```python
from build123d import *

# Parameters (mm, degrees)
SKETCH1_W           = 76.2
SKETCH1_H           = 9.525
SKETCH1_R           = 3.175
BOSS_EXTRUDE1_DEPTH = 12.7
CUT_EXTRUDE1_REACH  = 803.818
SKETCH2_R           = 2.6035


with BuildPart() as part:
    # Sketch1 → Boss-Extrude1 (new body)
    with BuildSketch(Plane(origin=(0, 788.156140976, 0), x_dir=(1, 0, 0), z_dir=(0, 1, 0))):
        with Locations((0, 58.7375)):
            Rectangle(SKETCH1_W, SKETCH1_H)
        with Locations(Location((-20.32, 58.7375, 0), (0, 0, 270))):
            Circle(SKETCH1_R, mode=Mode.SUBTRACT)
        with Locations(Location((20.32, 58.7375, 0), (0, 0, 90))):
            Circle(SKETCH1_R, mode=Mode.SUBTRACT)
    extrude(amount=BOSS_EXTRUDE1_DEPTH)

    # Sketch2 → Cut-Extrude1 (cut, up to next)
    with BuildSketch(Plane(origin=(0, 0, -63.5), x_dir=(-1, 0, 0), z_dir=(0, 0, -1)), mode=Mode.PRIVATE) as cut_extrude1_sk1:
        with Locations((30.1625, 794.506140976)):
            Circle(SKETCH2_R)
    cut_extrude1_tool1 = extrude(cut_extrude1_sk1.sketch, amount=-CUT_EXTRUDE1_REACH, mode=Mode.PRIVATE) & part.part
    # Sketch2 → Cut-Extrude1 (cut, up to next)
    with BuildSketch(Plane(origin=(0, 0, -63.5), x_dir=(-1, 0, 0), z_dir=(0, 0, -1)), mode=Mode.PRIVATE) as cut_extrude1_sk2:
        with Locations((-30.1625, 794.506140976)):
            Circle(SKETCH2_R)
    cut_extrude1_tool2 = extrude(cut_extrude1_sk2.sketch, amount=-CUT_EXTRUDE1_REACH, mode=Mode.PRIVATE) & part.part
    add(cut_extrude1_tool1.solids().sort_by_distance((-30.1625, 794.506141, -63.5))[0], mode=Mode.SUBTRACT)
    add(cut_extrude1_tool2.solids().sort_by_distance((30.1625, 794.506141, -63.5))[0], mode=Mode.SUBTRACT)


solid = part.part
```
Input: part model. Units: mm. Frame: model coordinates. Give positions to 0.01 mm unless a question says otherwise; leave off trailing zeros. Order: outer loops, then holes, each group sorted by start corner. A loop starts at its lowest first (then second) coordinate and runs counter-clockwise, first axis right, second up. Notation, with made-up numbers: (81.5, 64.25) - (91.5, 64.25) arc R26 ccw to (91.5, 92.25) - close; hole circle Ø3 at (51.5, -10.75). An arc over 180 degrees is marked (long way). Use a Markdown table: item, result.
(1) Line query: line 1 (X direction, y = 793.5, z = -56.5); line 2 (X direction, y = 795.75, z = -55); line 3 (X direction, y = 789.25, z = -61.25). Output: solid intervals per line, ascending. Write a range as from..to.
Computed values:
| item | result |
|---|---|
| line 1 | x = -38.1..-32.56, -27.76..-22.57, -18.07..18.07, 22.57..27.76, 32.56..38.1 |
| line 2 | x = -38.1..-32.45, -27.88..27.88, 32.45..38.1 |
| line 3 | x = -38.1..-22.26, -18.38..18.38, 22.26..38.1 |
(2) Pin query (flat end, axial travel): pin 1 (4 mm diameter, centred on x = 30.16, y = 794.51, fed in from +Z) (3 decimals). Return the tip coordinate at first contact, or that it passes through.
Computed values:
| item | result |
|---|---|
| pin 1 | passes through |
(3) Section query A-A (x = 20.32). Output: boundary loops of the cut face in (y, z) (1 decimal), then the cut area to 3 significant figures.
Computed values:
| item | result |
|---|---|
| outline | (788.2, -63.5) - (800.9, -63.5) - (800.9, -61.9) - (788.2, -61.9) - close; (788.2, -55.6) - (800.9, -55.6) - (800.9, -54) - (788.2, -54) - close |
| area | 40.3 mm2 |
(4) Draft query along Y for faces 1 (the flat face through (-1, 800.856, -59)), 2 (the cylindrical face through (30.727, 791.965, -58.804)), 3 (the flat face through (-38.1, 794, -59)). Return one class per face: released by +Y, released by -Y, zero draft, split by the parting line, or undercut.
Computed values:
| item | result |
|---|---|
| face 1 | released by +Y |
| face 2 | undercut |
| face 3 | zero draft |
(5) Section query B-B (z = -58.5). Output: boundary loops of the cut face in (x, y).
Computed values:
| item | result |
|---|---|
| outline | (-38.1, 788.16) - (-23.49, 788.16) - (-23.49, 800.86) - (-38.1, 800.86) - close; (-17.15, 788.16) - (17.15, 788.16) - (17.15, 800.86) - (-17.15, 800.86) - close; (23.49, 788.16) - (38.1, 788.16) - (38.1, 800.86) - (23.49, 800.86) - close; hole circle Ø5.21 at (-30.16, 794.51); hole circle Ø5.21 at (30.16, 794.51) |
(6) Section query C-C (y = 795.5). State how many separate pieces and enclosed holes the cut face has, then the cut area to 3 significant figures.
Computed values:
| item | result |
|---|---|
| separate pieces | 3 |
| enclosed holes | 2 |
| area | 571 mm2 |
